Read the model definition and answer for the solid it produces. Units are mm, in the model's axes. A direction names the side the tool comes from. Give positions to 0.01 mm unless a question says otherwise; leave off trailing zeros. Order: outer loops, then holes, each group sorted by start corner. A loop starts at its lowest first (then second) coordinate and runs counter-clockwise, first axis right, second up. Notation, with made-up numbers: M -21.75,-8 L -5.75,-8 A28 ccw -5.75,23 Z; hole C 32.25,28.5 d9. An arc over 180 degrees is marked long. One line per item, written item: value.
from build123d import *

# Parameters (mm, degrees)
BOSS_EXTRUDE1_DEPTH = 31.75
SKETCH2_R           = 3.302
CUT_EXTRUDE1_DEPTH  = 81.553334057
SKETCH3_R           = 3.302
CUT_EXTRUDE2_DEPTH  = 31.75
SKETCH4_R           = 3.302
CUT_EXTRUDE3_DEPTH  = 31.75
FILLET1_R           = 1.905
FILLET2_R           = 2.69875


with BuildPart() as part:
    # Sketch1 → Boss-Extrude1 (new body)
    with BuildSketch(Plane.XY):
        with BuildLine():
            Line((-17.009825212, -44.483777619), (-12.473871822, -32.621436921))
            ThreePointArc((-12.473871822, -32.621436921), (-34.344281252, 6.34239468), (0, 34.925))
            Line((0, 34.925), (42.249880176, 34.925))
            Line((42.249880176, 34.925), (42.249880176, 35.71875))
            Line((42.249880176, 35.71875), (0, 35.71875))
            ThreePointArc((0, 35.71875), (-35.050587448, 6.876439568), (-13.495614846, -33.071097373))
            Line((-13.495614846, -33.071097373), (-17.470874776, -43.467122992))
            ThreePointArc((-17.470874776, -43.467122992), (-64.678438716, -71.009375011), (-29.483697034, -112.82396454))
            Line((-29.483697034, -112.82396454), (22.258027731, -112.82396454))
            Line((22.258027731, -112.82396454), (22.258027731, -112.03021454))
            Line((22.258027731, -112.03021454), (-29.483697034, -112.03021454))
            ThreePointArc((-29.483697034, -112.03021454), (-63.827978286, -70.76281986), (-17.009825212, -44.483777619))
        make_face()
    extrude(amount=BOSS_EXTRUDE1_DEPTH)

    # Sketch2 → Cut-Extrude1 (cut, through all)
    with BuildSketch(Plane(origin=(-0.741396294, 0.283497087, 0), x_dir=(0, 0, 1), z_dir=(-0.934042575, 0.357161684, 0))):
        with Locations((7.9375, -41.275)):
            Circle(SKETCH2_R)
        with Locations((23.8125, -41.275)):
            Circle(SKETCH2_R)
    extrude(amount=-CUT_EXTRUDE1_DEPTH, mode=Mode.SUBTRACT)

    # Sketch3 → Cut-Extrude2 (cut)
    with BuildSketch(Plane(origin=(0, 35.71875, 0), x_dir=(1, 0, 0), z_dir=(0, 1, 0))):
        with Locations((34.925, -7.9375)):
            Circle(SKETCH3_R)
        with Locations((34.925, -23.8125)):
            Circle(SKETCH3_R)
    extrude(amount=-CUT_EXTRUDE2_DEPTH, mode=Mode.SUBTRACT)

    # Sketch4 → Cut-Extrude3 (cut)
    with BuildSketch(Plane.XZ.offset(112.82396454)):
        with Locations((5.441302966, 23.8125)):
            Circle(SKETCH4_R)
        with Locations((5.441302966, 7.9375)):
            Circle(SKETCH4_R)
    extrude(amount=-CUT_EXTRUDE3_DEPTH, mode=Mode.SUBTRACT)

    # Fillet1
    fillet1_edges = [part.edges().sort_by_distance(p)[0] for p in [
        (-17.470874776, -43.467122992, 15.875),
        (-13.495614846, -33.071097373, 15.875),
    ]]
    fillet(fillet1_edges, radius=FILLET1_R)

    # Fillet2
    fillet2_edges = [part.edges().sort_by_distance(p)[0] for p in [
        (-12.473871822, -32.621436921, 15.875),
        (-17.009825212, -44.483777619, 15.875),
    ]]
    fillet(fillet2_edges, radius=FILLET2_R)


solid = part.part
1) Find section A-A, the plane x = 20. Write down the section's boundary in (y, z) (3 decimals).
Reported:
outline: M -112.824,0 L -112.03,0 L -112.03,31.75 L -112.824,31.75 Z; M 34.925,0 L 35.719,0 L 35.719,31.75 L 34.925,31.75 Z
2) Consider probe 1 along Y at (x, z) = (11.5, 30) (3 decimals); probe 2 along Y at (x, z) = (-28, 29.5); probe 3 along Y at (x, z) = (-29, 23). Determine where each line is inside the solid, lowest interval first.
Reported:
probe 1: y = -112.824 to -112.03, 34.925 to 35.719
probe 2: y = -112.82 to -112.03, -42.21 to -41.42, -22.18 to -20.87, 20.87 to 22.18
probe 3: y = -112.82 to -112.03, -42.18 to -41.39, -20.85 to -19.46, 19.46 to 20.85
3) Find section C-C, the plane x = -24.5. Write down the section's boundary in (y, z), plus the area to 3 significant figures.
Reported:
outline: M -112.82,0 L -112.03,0 L -112.03,31.75 L -112.82,31.75 Z; M -42.54,0 L -41.74,0 L -41.74,31.75 L -42.54,31.75 Z; M -25.99,0 L -24.89,0 L -24.89,31.75 L -25.99,31.75 Z; M 24.89,0 L 25.99,0 L 25.99,31.75 L 24.89,31.75 Z
area: 121 mm^2
4) Find section B-B, the plane z = 22. Count the separate pieces of the cut face and the enclosed holes in it, plus the area to 3 significant figures.
Reported:
separate pieces: 4
enclosed holes: 0
area: 245 mm^2
5) Which of the six approach directions +Z, -Z, +X, -X, +Y, -Y give full straight-line access (tool end or side, diameter ignored) to faces 1 (the face through (-17.39, -43.5, 16.1)), 2 (the face through (-16.27, -41.42, 23.1)), 3 (the face through (4.73, -112.43, 20.59)), 4 (the face through (-14.76, -38.6, 15.65))?
Reported:
face 1: +Z, -Z
face 2: none
face 3: -Y
face 4: +Z, -Z, +X
6) Find section D-D, the plane y = -50.5. Write down the section's boundary in (x, z).
Reported:
outline: M -53.32,0 L -52.11,0 L -52.11,31.75 L -53.32,31.75 Z
7) Each of these flat-tipped pins is pushed along its axis until it touches: pin 1 Ø12 at (y, z) = (-42.5, 24.5) entering from +X; pin 2 Ø16 at (x, z) = (-16, 10) entering from +Y; pin 3 Ø4 at (x, z) = (34.92, 7.94) entering from -Y; pin 4 Ø5 at (x, z) = (-23, 15) entering from +Y. Where does it stop, or does it pass through?
Reported:
pin 1: stops at x = -14.1
pin 2: stops at y = 34.81
pin 3: passes through
pin 4: stops at y = 29.25
8) Determine the mould class of faces 5 (the face through (-64.146, -72.832, 15.653)), 6 (the face through (-16.27, -41.42, 7.22)) for opening direction Z: +Z half, -Z half, draft (parallel to the pull), parting line (faces both ways), or undercut.
Reported:
face 5: draft
face 6: undercut
